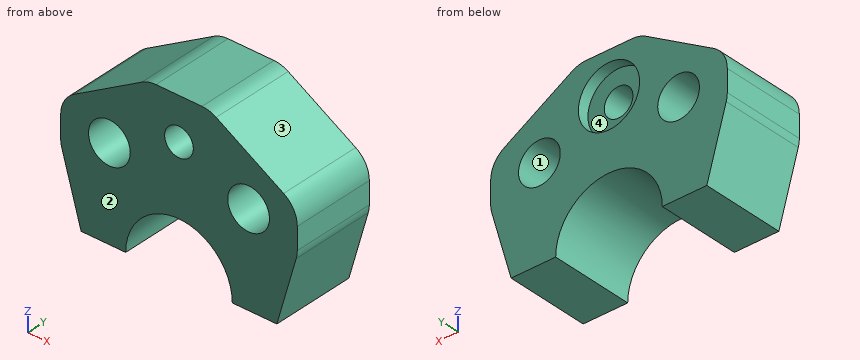
from build123d import *

# Parameters (mm, degrees)
SKETCH2_R           = 7.5
SKETCH2_R_2         = 5.15
BOSS_EXTRUDE1_DEPTH = 30
FILLET1_R           = 10
SKETCH4_R           = 11
CUT_EXTRUDE1_DEPTH  = 4


with BuildPart() as part:
    # Sketch2 → Boss-Extrude1 (new body)
    with BuildSketch(Plane(origin=(0, 0, 0), x_dir=(1, 0, 0), z_dir=(0, 1, 0))):
        with BuildLine():
            Line((35.15, 0), (19.15, 0))
            ThreePointArc((19.15, 0), (0, -19.15), (-19.15, 0))
            Line((-19.15, 0), (-35.15, 0))
            Line((-35.15, 0), (-42.5, -25.65))
            Line((-42.5, -25.65), (-42.5, -40.65))
            Line((-42.5, -40.65), (-11, -59.3))
            Line((-11, -59.3), (11, -59.3))
            Line((11, -59.3), (42.5, -40.65))
            Line((42.5, -40.65), (42.5, -25.65))
            Line((42.5, -25.65), (35.15, 0))
        make_face()
        with Locations((-25, -33.15)):
            Circle(SKETCH2_R, mode=Mode.SUBTRACT)
        with Locations((25, -33.15)):
            Circle(SKETCH2_R, mode=Mode.SUBTRACT)
        with Locations((0, -44.15)):
            Circle(SKETCH2_R_2, mode=Mode.SUBTRACT)
    extrude(amount=BOSS_EXTRUDE1_DEPTH)

    # Fillet1
    fillet1_edges = [part.edges().sort_by_distance(p)[0] for p in [
        (42.5, 15, 25.65),
        (42.5, 15, 40.65),
        (11, 15, 59.3),
        (-11, 15, 59.3),
        (-42.5, 15, 40.65),
        (-42.5, 15, 25.65),
    ]]
    fillet(fillet1_edges, radius=FILLET1_R)

    # Sketch4 → Cut-Extrude1 (cut)
    with BuildSketch(Plane(origin=(0, 30, 0), x_dir=(1, 0, 0), z_dir=(0, 1, 0))):
        with Locations((0, -44.15)):
            Circle(SKETCH4_R)
    extrude(amount=-CUT_EXTRUDE1_DEPTH, mode=Mode.SUBTRACT)


solid = part.part
Verification items for the finished model (mm, model axes). Face numbers are marked on the shaded views. Give positions to 0.01 mm unless a question says otherwise; leave off trailing zeros. Loops run counter-clockwise (first coordinate to the right, second up) from the corner with the lowest first, then second, coordinate; pieces in that order, holes last.
1. Cross-section at A-A on x = 0. Record the cut outline in (y, z).
Derived:
outline: (0, 19.15) - (30, 19.15) - (30, 33.15) - (26, 33.15) - (26, 39) - (0, 39) - close; (0, 49.3) - (26, 49.3) - (26, 55.15) - (30, 55.15) - (30, 59.3) - (0, 59.3) - close
2. Release check for a two-part mould opening along X. For the marked faces 1, 2, 3 and 4 record: +X half, -X half, draft (parallel to the pull), parting line (faces both ways), or undercut.
Derived:
face 1: undercut
face 2: draft
face 3: +X half
face 4: undercut
3. Cross-section at D-D on z = 17. Record the cut outline in (x, y).
Derived:
outline: (-40.02, 0) - (-8.82, 0) - (-8.82, 30) - (-40.02, 30) - close; (8.82, 0) - (40.02, 0) - (40.02, 30) - (8.82, 30) - close
4. Cross-section at B-B on y = 27.75. Record the cut outline in (x, z), and give its area (3 significant figures).
Derived:
outline: (-42.5, 27.05) arc R10 ccw to (-42.11, 24.3) - (-35.15, 0) - (-19.15, 0) arc R19.15 cw to (19.15, 0) - (35.15, 0) - (42.11, 24.3) arc R10 ccw to (42.5, 27.05) - (42.5, 34.95) arc R10 ccw to (37.59, 43.55) - (13.36, 57.9) arc R10 ccw to (8.26, 59.3) - (-8.26, 59.3) arc R10 ccw to (-13.36, 57.9) - (-37.59, 43.55) arc R10 ccw to (-42.5, 34.95) - close; hole circle Ø15 at (-25, 33.15); hole circle Ø22 at (0, 44.15); hole circle Ø15 at (25, 33.15)
area: 2,940 mm2
5. Cross-section at C-C on z = 29. Record the cut outline in (x, y).
Derived:
outline: (-42.5, 0) - (-31.25, 0) - (-31.25, 30) - (-42.5, 30) - close; (-18.75, 0) - (18.75, 0) - (18.75, 30) - (-18.75, 30) - close; (31.25, 0) - (42.5, 0) - (42.5, 30) - (31.25, 30) - close
6. Material ranges on probe 1 along X at (y, z) = (7, 33); probe 2 along Z at (x, y) = (0, 27); probe 3 along Z at (x, y) = (0, 17), recorded low to high.
Derived:
probe 1: x = -42.5 to -32.5, -17.5 to 17.5, 32.5 to 42.5
probe 2: z = 19.15 to 33.15, 55.15 to 59.3
probe 3: z = 19.15 to 39, 49.3 to 59.3
7. Go/stop test with flat-tipped pins: P1, Ø1.5, axis at y = 13, z = 6.5, coming from the -X side; P2, Ø6.5, axis at x = -4.5, z = 47.5, coming from the +Y side; P3, Ø8, axis at y = 12.5, z = 51, coming from the -X side. Record where each tip stops, or that it passes through.
Derived:
P1: stops at x = -37.23
P2: stops at y = 26
P3: stops at x = -31.77
